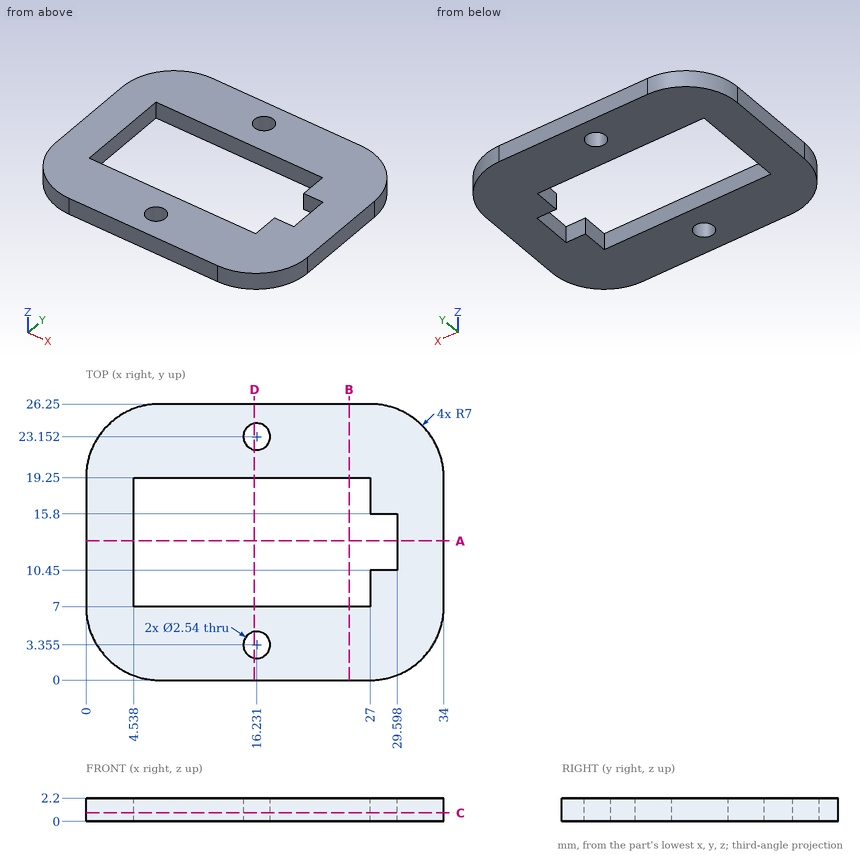
Job drawing, mm, ordinate dimensions from the low corner. One solid piece. Coordinates: 2 decimals unless noted, no trailing zeros. Loops run counter-clockwise (first coordinate to the right, second up) from the corner with the lowest first, then second, coordinate; pieces in that order, holes last. Notation, with made-up numbers: (-18.75, -2) -> (27.25, -2) arc R20 cw to (27.25, 35) -> close; hole circle Ø11 at (37, 28). An arc over 180 degrees is marked (long way). One line per item, written item: value.
1. Slice it at A-A on y = 13.25. Write the cut outline in (x, z).
Answers:
outline: (0, 0) -> (4.54, 0) -> (4.54, 2.2) -> (0, 2.2) -> close; (29.6, 0) -> (34, 0) -> (34, 2.2) -> (29.6, 2.2) -> close
2. Flat gauge pin, fed straight in: P1, Ø1.5, axis at x = 16.23, y = 3.36, coming from the +Z side. Where does the tip first touch, or does it go through?
Answers:
P1: passes through
3. Slice it at B-B on x = 25. Write the cut outline in (y, z).
Answers:
outline: (0, 0) -> (7, 0) -> (7, 2.2) -> (0, 2.2) -> close; (19.25, 0) -> (26.25, 0) -> (26.25, 2.2) -> (19.25, 2.2) -> close
4. Drill centre lines: line 1 (Y direction, x = 26.5, z = 0.5); line 2 (X direction, y = 15.75, z = 0.75); line 3 (X direction, y = 9.25, z = 1.5). Where is each one in solid material? Low to high. Write a range as [from, to].
Answers:
line 1: y = [0, 7], [19.25, 26.25]
line 2: x = [0, 4.54], [29.6, 34]
line 3: x = [0, 4.54], [27, 34]
5. Slice it at D-D on x = 16. Write the cut outline in (y, z), and give its area (3 significant figures).
Answers:
outline: (0, 0) -> (2.11, 0) -> (2.11, 2.2) -> (0, 2.2) -> close; (4.6, 0) -> (7, 0) -> (7, 2.2) -> (4.6, 2.2) -> close; (19.25, 0) -> (21.9, 0) -> (21.9, 2.2) -> (19.25, 2.2) -> close; (24.4, 0) -> (26.25, 0) -> (26.25, 2.2) -> (24.4, 2.2) -> close
area: 19.8 mm^2
6. Slice it at C-C on z = 0.8. Give the number of separate pieces and of enclosed holes in the cut face, and give its area (3 significant figures).
Answers:
separate pieces: 1
enclosed holes: 3
area: 551 mm^2
